Geometry: final body of the model. Coordinates: model frame, mm. Give positions to 0.01 mm unless a question says otherwise; leave off trailing zeros. Loops run counter-clockwise (first coordinate to the right, second up) from the corner with the lowest first, then second, coordinate; pieces in that order, holes last.
from build123d import *

# Parameters (mm, degrees)
F0_W     = 10.5
F0_H     = 127
F1_ANGLE = 180
F3_DEPTH = 127
F4_R     = 1
F5_R     = 1


with BuildPart() as f1:
    # F0 (on Front) → F1 (revolve)
    with BuildSketch(Plane.XZ):
        Rectangle(F0_W, F0_H)
    revolve(axis=Axis((5.25, 0, 0), (0, 0, -1)), revolution_arc=F1_ANGLE)

    # F2 (on face) → F3 (cut)
    with BuildSketch(Plane.XY.offset(63.5)):
        with BuildLine():
            Line((-0.75, 0), (5.25, 0))
            Line((5.25, 0), (11.25, 0))
            Line((11.25, 0), (11.25, 1.8))
            ThreePointArc((11.25, 1.8), (11.1914213562, 1.9414213562), (11.05, 2))
            Line((11.05, 2), (-0.55, 2))
            ThreePointArc((-0.55, 2), (-0.6914213562, 1.9414213562), (-0.75, 1.8))
            Line((-0.75, 1.8), (-0.75, 0))
        make_face()
    extrude(amount=-F3_DEPTH, mode=Mode.SUBTRACT)

    # F4
    f4_edges = [f1.edges().sort_by_distance(p)[0] for p in [
        (5.25, 10.5, 63.5),
    ]]
    fillet(f4_edges, radius=F4_R)

    # F5
    f5_edges = [f1.edges().sort_by_distance(p)[0] for p in [
        (5.25, 10.5, -63.5),
    ]]
    fillet(f5_edges, radius=F5_R)


with BuildPart() as f6_1:
    # F6: instance of F1
    add(f1.part.mirror(Plane.XZ))


solid = f6_1.part
Item 1: Pin query (flat end, axial travel): pin 1 (5 mm diameter, centred on x = -1.5, z = -12.5, fed in from -Y); pin 2 (2 mm diameter, centred on y = -2.5, z = 47, fed in from -X); pin 3 (0.9 mm diameter, centred on y = -1, z = 8, fed in from +X); pin 4 (6 mm diameter, centred on x = 7, z = 49.5, fed in from -Y). Return the tip coordinate at first contact, or that it passes through.
Values follow:
pin 1: stops at y = -9.6
pin 2: stops at x = -5.14
pin 3: stops at x = 15.74
pin 4: stops at y = -10.5
Item 2: Ray query, probe 1 along Y at (x, z) = (4.75, -43.5); probe 2 along X at (y, z) = (-4.5, -6.5); probe 3 along X at (y, z) = (-1.5, -23.5). Return the intervals inside material, ascending.
Values follow:
probe 1: y = -10.49 to -2
probe 2: x = -4.24 to 14.74
probe 3: x = -5.14 to -0.75, 11.25 to 15.64
Item 3: Draft query along X for faces 1 (the face through (5, -5, -63.5)), 2 (the face through (5, -2, 1)), 3 (the face through (5.019, -10.497, 0.875)). Return one class per face: +X half, -X half, draft (parallel to the pull), parting line (faces both ways), or undercut.
Values follow:
face 1: draft
face 2: undercut
face 3: parting line
Item 4: Section query A-A on z = 45. Return loops of the section in (x, y), plus the area to 3 significant figures.
Values follow:
outline: (-5.25, 0) arc R10.5 ccw to (15.75, 0) - (11.25, 0) - (11.25, -1.8) arc R0.2 cw to (11.05, -2) - (-0.55, -2) arc R0.2 cw to (-0.75, -1.8) - (-0.75, 0) - close
area: 149 mm2
Item 5: Section query B-B on x = 5.25. Return loops of the section in (y, z).
Values follow:
outline: (-10.5, -62.5) arc R1 ccw to (-9.5, -63.5) - (-2, -63.5) - (-2, 63.5) - (-9.5, 63.5) arc R1 ccw to (-10.5, 62.5) - close
